Can you work these out from the model? Positions are in its coordinate system, mm. A direction names the side the tool comes from. Give positions to 0.01 mm unless a question says otherwise; leave off trailing zeros. Loops run counter-clockwise (first coordinate to the right, second up) from the corner with the lowest first, then second, coordinate; pieces in that order, holes last. Notation, with made-up numbers: (24.5, -20) - (34.5, -20) arc R35 ccw to (34.5, 15) - close; hole circle Ø10 at (34, 82.25). An arc over 180 degrees is marked (long way). Answer in a Markdown table with one row per item.
from build123d import *
from build123d import SkipClean  # not in build123d's __all__

# Parameters (mm, degrees)
F0_R     = 118.5
F1_DEPTH = 20
F2_DEPTH = 20
F4_DEPTH = 4
F6_DEPTH = 4


with BuildPart() as f1:
    # F0 (on Top) → F1 (new body)
    with BuildSketch(Plane.XY):
        Circle(F0_R)
        with BuildLine():
            ThreePointArc((84.4585554209, 26.4386538277), (87.4838046576, 13.3728801171), (88.5, 0))
            ThreePointArc((88.5, 0), (76.2236705877, -44.9689008331), (42.8005188217, -77.4620267524))
            ThreePointArc((42.8005188217, -77.4620267524), (33.7736370968, -81.8021481213), (24.3141576643, -85.0944871133))
            ThreePointArc((24.3141576643, -85.0944871133), (-1.1327702213, -88.4927501642), (-26.4843739752, -84.4442297327))
            ThreePointArc((-26.4843739752, -84.4442297327), (-35.8564791301, -80.9108330472), (-44.7693079971, -76.3410706072))
            ThreePointArc((-44.7693079971, -76.3410706072), (-82.6573501675, -31.6229736629), (-84.2920148647, 26.9649073806))
            ThreePointArc((-84.2920148647, 26.9649073806), (-79.5306754268, 38.821664907), (-73.1116226226, 49.869235381))
            ThreePointArc((-73.1116226226, 49.869235381), (-59.6374598942, 65.3882510652), (-42.9470514929, 77.3808811533))
            ThreePointArc((-42.9470514929, 77.3808811533), (-33.9284003129, 81.7380795726), (-24.4751691036, 85.0483162523))
            ThreePointArc((-24.4751691036, 85.0483162523), (0.6651888823, 88.4975000989), (25.7508578518, 84.6707937833))
            ThreePointArc((25.7508578518, 84.6707937833), (35.1532611727, 81.2188292758), (44.1053955412, 76.7265539703))
            ThreePointArc((44.1053955412, 76.7265539703), (60.8748593955, 64.2378509414), (74.2463940977, 48.1635024005))
            ThreePointArc((74.2463940977, 48.1635024005), (80.0924934797, 37.6489374113), (84.4585554209, 26.4386538277))
        make_face(mode=Mode.SUBTRACT)
    extrude(amount=F1_DEPTH)

    # F0 (on Top) → F2 (join)
    with BuildSketch(Plane.XY):
        with BuildLine():
            Line((-84.2920148647, 26.9649073806), (-44.7693079971, -76.3410706072))
            Line((-44.7693079971, -76.3410706072), (-33.3414858158, -50.5729274495))
            Line((-33.3414858158, -50.5729274495), (-73.1116226226, 49.869235381))
            ThreePointArc((-73.1116226226, 49.869235381), (-79.5306754268, 38.821664907), (-84.2920148647, 26.9649073806))
        make_face()
        with BuildLine():
            ThreePointArc((-44.7693079971, -76.3410706072), (-35.8564791301, -80.9108330472), (-26.4843739752, -84.4442297327))
            Line((-26.4843739752, -84.4442297327), (-0.5078915586, -25.1346434059))
            Line((-0.5078915586, -25.1346434059), (-10.9130780509, 0))
            Line((-10.9130780509, 0), (-33.3414858158, -50.5729274495))
            Line((-33.3414858158, -50.5729274495), (-44.7693079971, -76.3410706072))
        make_face()
        with BuildLine():
            Line((9.6563450565, -1.9276264085), (44.1053955412, 76.7265539703))
            ThreePointArc((44.1053955412, 76.7265539703), (35.1532611727, 81.2188292758), (25.7508578518, 84.6707937833))
            Line((25.7508578518, 84.6707937833), (0, 20.3185360879))
            Line((0, 20.3185360879), (-24.4751691036, 85.0483162523))
            ThreePointArc((-24.4751691036, 85.0483162523), (-33.9284003129, 81.7380795726), (-42.9470514929, 77.3808811533))
            Line((-42.9470514929, 77.3808811533), (-10.9130780509, 0))
            Line((-10.9130780509, 0), (-0.5078915586, -25.1346434059))
            Line((-0.5078915586, -25.1346434059), (9.6563450565, -1.9276264085))
        make_face()
        with BuildLine():
            ThreePointArc((24.3141576643, -85.0944871133), (33.7736370968, -81.8021481213), (42.8005188217, -77.4620267524))
            Line((42.8005188217, -77.4620267524), (31.0016963563, -50.5729274495))
            Line((31.0016963563, -50.5729274495), (9.6563450565, -1.9276264085))
            Line((9.6563450565, -1.9276264085), (-0.5078915586, -25.1346434059))
            Line((-0.5078915586, -25.1346434059), (24.3141576643, -85.0944871133))
        make_face()
        with BuildLine():
            Line((42.8005188217, -77.4620267524), (84.4585554209, 26.4386538277))
            ThreePointArc((84.4585554209, 26.4386538277), (80.0924934797, 37.6489374113), (74.2463940977, 48.1635024005))
            Line((74.2463940977, 48.1635024005), (31.0016963563, -50.5729274495))
            Line((31.0016963563, -50.5729274495), (42.8005188217, -77.4620267524))
        make_face()
    extrude(amount=F2_DEPTH)

    # F3 (on face) → F4 (cut)
    with BuildSketch(Plane.XY.offset(20)):
        with BuildLine():
            ThreePointArc((24.3141576643, -85.0944871133), (33.7736370968, -81.8021481213), (42.8005188217, -77.4620267524))
            Line((42.8005188217, -77.4620267524), (45.8884559448, -69.7603011103))
            ThreePointArc((45.8884559448, -69.7603011103), (34.5537158667, -76.0150690311), (22.3883760006, -80.4425920769))
            Line((22.3883760006, -80.4425920769), (24.3141576643, -85.0944871133))
        make_face()
        with BuildLine():
            ThreePointArc((-44.7693079971, -76.3410706072), (-35.8564791301, -80.9108330472), (-26.4843739752, -84.4442297327))
            Line((-26.4843739752, -84.4442297327), (-24.4657542833, -79.8353109053))
            ThreePointArc((-24.4657542833, -79.8353109053), (-36.5644517119, -75.068574457), (-47.7763395541, -68.4811753609))
            Line((-47.7763395541, -68.4811753609), (-44.7693079971, -76.3410706072))
        make_face()
        with BuildLine():
            ThreePointArc((-73.1116226226, 49.869235381), (-79.5306754268, 38.821664907), (-84.2920148647, 26.9649073806))
            Line((-84.2920148647, 26.9649073806), (-81.2849833078, 19.1050121343))
            ThreePointArc((-81.2849833078, 19.1050121343), (-77.0970321509, 32.067080215), (-70.8572793817, 44.1757394803))
            Line((-70.8572793817, 44.1757394803), (-73.1116226226, 49.869235381))
        make_face()
        with BuildLine():
            Line((-22.7005830367, 80.3550466977), (-24.4751691036, 85.0483162523))
            ThreePointArc((-24.4751691036, 85.0483162523), (-33.9284003129, 81.7380795726), (-42.9470514929, 77.3808811533))
            Line((-42.9470514929, 77.3808811533), (-41.0212698292, 72.728986117))
            ThreePointArc((-41.0212698292, 72.728986117), (-32.0882818667, 77.0882102973), (-22.7005830367, 80.3550466977))
        make_face()
        with BuildLine():
            Line((42.0867758493, 72.117635143), (44.1053955412, 76.7265539703))
            ThreePointArc((44.1053955412, 76.7265539703), (35.1532611727, 81.2188292758), (25.7508578518, 84.6707937833))
            Line((25.7508578518, 84.6707937833), (23.8860818979, 80.0106561126))
            ThreePointArc((23.8860818979, 80.0106561126), (33.2216711626, 76.6065960943), (42.0867758493, 72.117635143))
        make_face()
        with BuildLine():
            Line((81.3706182978, 18.7369281856), (84.4585554209, 26.4386538277))
            ThreePointArc((84.4585554209, 26.4386538277), (80.0924934797, 37.6489374113), (74.2463940977, 48.1635024005))
            Line((74.2463940977, 48.1635024005), (71.8122254689, 42.6058009338))
            ThreePointArc((71.8122254689, 42.6058009338), (77.515654404, 31.0414774507), (81.3706182978, 18.7369281856))
        make_face()
    with SkipClean():  # cleaning this boolean's faces spoils the solid; the shape is the same uncleaned
        extrude(amount=-F4_DEPTH, mode=Mode.SUBTRACT)

    # F5 (on face) → F6 (cut)
    with BuildSketch(Plane(origin=(0, 0, 0), x_dir=(1, 0, 0), z_dir=(0, 0, -1))):
        with BuildLine():
            Line((-24.4657542833, 79.8353109053), (-26.4843739752, 84.4442297327))
            ThreePointArc((-26.4843739752, 84.4442297327), (-35.8564791301, 80.9108330472), (-44.7693079971, 76.3410706072))
            Line((-44.7693079971, 76.3410706072), (-47.7763395541, 68.4811753609))
            ThreePointArc((-47.7763395541, 68.4811753609), (-36.5644517119, 75.068574457), (-24.4657542833, 79.8353109053))
        make_face()
        with BuildLine():
            Line((45.8884559448, 69.7603011104), (42.8005188217, 77.4620267524))
            ThreePointArc((42.8005188217, 77.4620267524), (33.7736370968, 81.8021481213), (24.3141576643, 85.0944871133))
            Line((24.3141576643, 85.0944871133), (22.3883760006, 80.4425920769))
            ThreePointArc((22.3883760006, 80.4425920769), (34.5537158667, 76.0150690311), (45.8884559448, 69.7603011103))
        make_face()
        with BuildLine():
            ThreePointArc((74.2463940977, -48.1635024005), (80.0924934797, -37.6489374113), (84.4585554209, -26.4386538277))
            Line((84.4585554209, -26.4386538277), (81.3706182978, -18.7369281856))
            ThreePointArc((81.3706182978, -18.7369281856), (77.515654404, -31.0414774507), (71.8122254689, -42.6058009338))
            Line((71.8122254689, -42.6058009338), (74.2463940977, -48.1635024005))
        make_face()
        with BuildLine():
            ThreePointArc((25.7508578518, -84.6707937833), (35.1532611727, -81.2188292758), (44.1053955412, -76.7265539703))
            Line((44.1053955412, -76.7265539703), (42.0867758493, -72.117635143))
            ThreePointArc((42.0867758493, -72.117635143), (33.2216711626, -76.6065960943), (23.8860818979, -80.0106561126))
            Line((23.8860818979, -80.0106561126), (25.7508578518, -84.6707937833))
        make_face()
        with BuildLine():
            ThreePointArc((-42.9470514929, -77.3808811533), (-33.9284003129, -81.7380795726), (-24.4751691036, -85.0483162523))
            Line((-24.4751691036, -85.0483162523), (-22.7005830367, -80.3550466977))
            ThreePointArc((-22.7005830367, -80.3550466977), (-32.0882818667, -77.0882102973), (-41.0212698292, -72.728986117))
            Line((-41.0212698292, -72.728986117), (-42.9470514929, -77.3808811533))
        make_face()
        with BuildLine():
            Line((-81.2849833078, -19.1050121343), (-84.2920148647, -26.9649073806))
            ThreePointArc((-84.2920148647, -26.9649073806), (-79.5306754268, -38.821664907), (-73.1116226226, -49.869235381))
            Line((-73.1116226226, -49.869235381), (-70.8572793817, -44.1757394803))
            ThreePointArc((-70.8572793817, -44.1757394803), (-77.0970321509, -32.067080215), (-81.2849833078, -19.1050121343))
        make_face()
    extrude(amount=-F6_DEPTH, mode=Mode.SUBTRACT)


solid = f1.part
Q1. Imagine slicing it at C-C, the plane y = -37.5. Write out the boundary of the cut face in (x, z).
Checked values:
| item | result |
|---|---|
| outline | (-112.41, 0) - (-80.16, 0) - (-80.16, 20) - (-112.41, 20) - close; (-59.63, 0) - (-38.52, 0) - (-38.52, 20) - (-59.63, 20) - close; (-27.54, 0) - (-5.92, 0) - (-5.92, 20) - (-27.54, 20) - close; (4.61, 0) - (25.27, 0) - (25.27, 20) - (4.61, 20) - close; (36.73, 0) - (58.82, 0) - (58.82, 20) - (36.73, 20) - close; (80.16, 0) - (112.41, 0) - (112.41, 20) - (80.16, 20) - close |
Q2. For pin 1 (5 mm diameter, centred on x = 61, z = 13.5, fed in from -Y); pin 2 (4 mm diameter, centred on y = -46.5, z = 15.5, fed in from +X); pin 3 (1.5 mm diameter, centred on x = 21.5, z = 16.5, fed in from +Y), each with a flat end and sliding along its axis, tell me the tip position at first contact or that it passes through.
Checked values:
| item | result |
|---|---|
| pin 1 | stops at y = -103.05 |
| pin 2 | stops at x = 109.83 |
| pin 3 | stops at y = 116.67 |
Q3. Imagine slicing it at B-B, the plane x = -36.5. Write out the boundary of the cut face in (y, z).
Checked values:
| item | result |
|---|---|
| outline | (-112.74, 0) - (-80.62, 0) - (-80.62, 4) - (-75.1, 4) - (-75.1, 0) - (-42.6, 0) - (-42.6, 20) - (-75.1, 20) - (-75.1, 16) - (-80.62, 16) - (-80.62, 20) - (-112.74, 20) - close; (61.81, 0) - (75.1, 0) - (75.1, 4) - (80.62, 4) - (80.62, 0) - (112.74, 0) - (112.74, 20) - (80.62, 20) - (80.62, 16) - (75.1, 16) - (75.1, 20) - (61.81, 20) - close |
Q4. If we mould it in two halves opening along Y, with no side actions, what happens to faces 5 (the face through (0, 0, 20)), 6 (the face through (-118.385, 5.21, 9.86)), 7 (the face through (13.056, 52.945, 9.86))? For each: released by +Y, released by -Y, zero draft, split by the parting line, or undercut.
Checked values:
| item | result |
|---|---|
| face 5 | zero draft |
| face 6 | split by the parting line |
| face 7 | undercut |
Q5. Imagine slicing it at A-A, the plane y = -10. Write out the boundary of the cut face in (x, z), and give its area (3 significant figures).
Checked values:
| item | result |
|---|---|
| outline | (-118.08, 0) - (-87.93, 0) - (-87.93, 20) - (-118.08, 20) - close; (-70.15, 0) - (-49.41, 0) - (-49.41, 20) - (-70.15, 20) - close; (-15.35, 0) - (13.2, 0) - (13.2, 20) - (-15.35, 20) - close; (48.77, 0) - (69.85, 0) - (69.85, 20) - (48.77, 20) - close; (87.93, 0) - (118.08, 0) - (118.08, 20) - (87.93, 20) - close |
| area | 2,610 mm² |
Q6. If I drill on line 1 (X direction, y = 33.5, z = 14.25); line 2 (X direction, y = -54.5, z = 17.25); line 3 (X direction, y = -4, z = 9), over which ranges is the centre line in solid material (lowest first)? Write a range as [from, to].
Checked values:
| item | result |
|---|---|
| line 1 | x = [-113.67, -66.63], [-24.78, -4.98], [5.27, 25.17], [67.82, 113.67] |
| line 2 | x = [-105.22, -69.73], [-53.13, -13.37], [11.65, 52.01], [69.73, 105.22] |
| line 3 | x = [-118.43, -88.41], [-72.45, -51.78], [-12.69, 10.57], [51.4, 72.25], [88.41, 118.43] |
Q7. On a 3-axis mill with a long thin cutter (end or side, diameter ignored), from which of +Z, -Z, +X, -X, +Y, -Y can I reach the whole of each face in a straight line? I mean faces 1 (the face through (0, 0, 0)), 2 (the face through (-36.4, -75.15, 18.03)), 3 (the face through (-36, -76, 4)), 4 (the face through (26.64, 36.85, 9.86)). Say none if no direction works.
Checked values:
| item | result |
|---|---|
| face 1 | -Z, +X, -X, +Y, -Y |
| face 2 | +Z |
| face 3 | -Z |
| face 4 | +Z, -Z |
Q8. Imagine slicing it at D-D, the plane y = 15. Write out the boundary of the cut face in (x, z).
Checked values:
| item | result |
|---|---|
| outline | (-117.55, 0) - (-87.22, 0) - (-87.22, 20) - (-117.55, 20) - close; (-79.71, 0) - (-59.31, 0) - (-59.31, 20) - (-79.71, 20) - close; (-17.12, 0) - (17.07, 0) - (17.07, 20) - (-17.12, 20) - close; (59.72, 0) - (79.87, 0) - (79.87, 20) - (59.72, 20) - close; (87.22, 0) - (117.55, 0) - (117.55, 20) - (87.22, 20) - close |
